The drawing under review shows one solid part. Ordinate dimensions are in mm from its lowest x, y, z. A direction names the side the tool comes from. Round coordinates to 2 decimals unless told otherwise and drop trailing zeros. Order: outer loops, then holes, each group sorted by start corner. A loop starts at its lowest first (then second) coordinate and runs counter-clockwise, first axis right, second up.
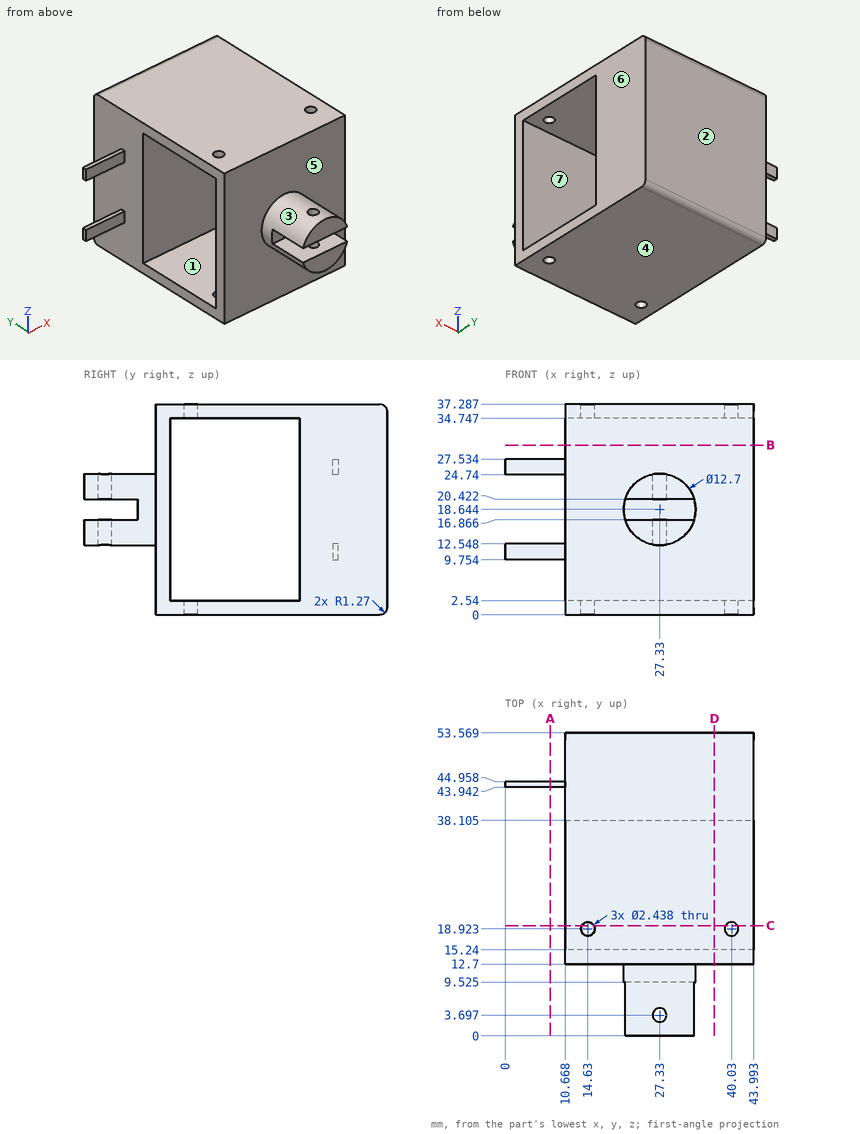
Q1. Clearance check with flat-ended pins moving along their axes: pin 1 (0.8 mm diameter, centred on x = 7, z = 26.5, fed in from +Y); pin 2 (10 mm diameter, centred on x = 29.5, z = 33.5, fed in from -Y); pin 3 (1.1 mm diameter, centred on x = 7.5, y = 44.5, fed in from +Z). State where each tip first meets the part, or that it passes through.
Q2. Take a section at A-A, the plane x = 8. State the section outline as (y, z) points.
Q3. Tool access review of the marked faces 5, 6 and 7: name each direction out of +Z, -Z, +X, -X, +Y, -Y from which nothing blocks a thin tool from reaching the whole face with its end or side.
Q4. Mouldability with a two-part tool opening along Z and no side actions: class the marked faces 1, 2, 3 and 4 as +Z half, -Z half, draft (parallel to the pull), parting line (faces both ways), or undercut.
Q5. Wall thickness on line 1 (Y direction, x = 21, z = 31.5) (1 decimal); line 2 (Z direction, x = 13.5, y = 20); line 3 (Y direction, x = 28, z = 16) (1 decimal): over which ranges is each line inside the solid? List them lowest first.
Q6. Take a section at B-B, the plane z = 30. State the section outline as (x, y) points (1 decimal).
Q7. Take a section at C-C, the plane y = 19.5. State the section outline as (x, z) points (1 decimal).
Q8. Take a section at D-D, the plane x = 37. State the section outline as (y, z) points (1 decimal).
Working result:
1. pin 1: stops at y = 44.96
1. pin 2: stops at y = 12.7
1. pin 3: stops at z = 27.53
2. outline: (43.94, 9.75) - (44.96, 9.75) - (44.96, 12.55) - (43.94, 12.55) - close; (43.94, 24.74) - (44.96, 24.74) - (44.96, 27.53) - (43.94, 27.53) - close
3. face 5: -Y
3. face 6: +Z, -Z, +X, +Y, -Y
3. face 7: +X, -X
4. face 1: undercut
4. face 2: draft
4. face 3: parting line
4. face 4: -Z half
5. line 1: y = 12.7 to 15.2, 38.1 to 53.6
5. line 2: z = 0 to 2.54, 34.75 to 37.29
5. line 3: y = 0 to 2.7, 4.7 to 15.2, 38.1 to 53.6
6. outline: (10.7, 12.7) - (44, 12.7) - (44, 15.2) - (10.7, 15.2) - close; (10.7, 38.1) - (44, 38.1) - (44, 53.6) - (10.7, 53.6) - close
7. outline: (10.7, 0) - (13.6, 0) - (13.6, 2.5) - (10.7, 2.5) - close; (10.7, 34.7) - (13.6, 34.7) - (13.6, 37.3) - (10.7, 37.3) - close; (15.7, 0) - (39, 0) - (39, 2.5) - (15.7, 2.5) - close; (15.7, 34.7) - (39, 34.7) - (39, 37.3) - (15.7, 37.3) - close; (41.1, 0) - (44, 0) - (44, 2.5) - (41.1, 2.5) - close; (41.1, 34.7) - (44, 34.7) - (44, 37.3) - (41.1, 37.3) - close
8. outline: (12.7, 0) - (52.3, 0) arc R1.3 ccw to (53.6, 1.3) - (53.6, 36) arc R1.3 ccw to (52.3, 37.3) - (12.7, 37.3) - close; hole (15.2, 2.5) - (38.1, 2.5) - (38.1, 34.7) - (15.2, 34.7) - close
